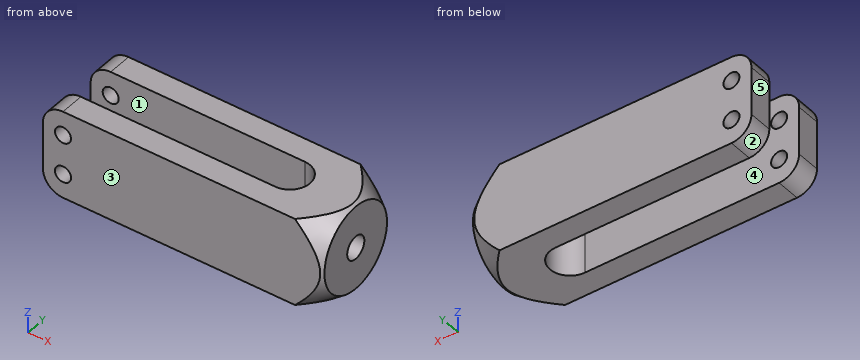
Autodesk Inventor part; units mm, degrees
ref_plane "Work Plane1" through (111.125, 34.925, 0) normal (0, 0.7071, 0.7071) x (-1, 0, 0)
ref_plane "YZ Plane" through (0, 0, 0) normal (1, 0, 0) x (0, 1, 0)
ref_plane "XZ Plane" through (0, 0, 0) normal (0, 1, 0) x (-1, 0, 0)
sketch "Sketch1" plane through (0, 0, 0) normal (0, 0, 1) x (1, 0, 0)
  line L0 (0, 0) -> (111.125, 0)
  line L1 (111.125, 0) -> (111.125, 34.925)
  line L2 (111.125, 34.925) -> (0, 34.925)
  arc A0 (85.0138, 9.525) -> (85.0138, 25.4) centre (85.0138, 17.4625) ccw
  line L3 (85.0138, 25.4) -> (0, 25.4)
  line L4 (0, 9.525) -> (85.0138, 9.525)
  line L5 (85.0138, 9.525) -> (85.0138, 25.4)
  line L6 (0, 34.925) -> (0, 25.4)
  line L7 (0, 9.525) -> (0, 0)
  dimension "d0" = 34.925
  dimension "d2" = 15.875
  dimension "d3" = 85.0138
  dimension "d4" = 111.125
extrude "Extrusion1" add sketch "Sketch1" along normal blind 34.925 contours L7 L4 A0 L3 L6 L2 L1 L0
sketch "Sketch2" plane through (111.125, 0, 0) normal (1, 0, 0) x (0, 0, -1)
  point P0 (0, 0)
  point P1 (-17.4625, 17.4752)
hole "Hole1" at (111.125, 17.4752, 17.4625) direction (-1, 0, 0) diameter 9.144 end through all
ref_plane "Work Plane1" through (111.125, 34.925, 0) normal (0, 0.7071, 0.7071) x (-1, 0, 0)
sketch "Sketch3" plane through (111.125, 34.925, 0) normal (0, 0.7071, 0.7071) x (-1, 0, 0)
  line L0 (0, 0) -> (111.125, 0)
  line L1 (111.125, 0) -> (111.125, 24.6957)
  line L2 (0, 24.6957) -> (111.125, 24.6957)
  line L3 (0, 0) -> (0, 24.6957)
  line L4 (0, 0) -> (0, 24.6957)
  line L5 (0, 8.027) -> (11.1125, 0)
  line L6 (11.1125, 0) -> (0, 0)
  line L7 (0, 8.027) -> (0, 0)
  dimension "d14" = 11.1125
  dimension "d15" = 16.6687
revolve "Revolution1" cut sketch "Sketch3" angle 360 about axis through (111.125, 17.4625, 17.4625) along (-1, 0, 0) contours L3 L5 L0
fillet "Fillet1" radius 7.9375 4 edges at (0, 30.1625, 0) (0, 4.7625, 0) (0, 4.7625, 34.925) (0, 30.1625, 34.925)
sketch "Sketch4" plane through (7.9375, 0, 0) normal (0, -1, 0) x (1, 0, 0)
  point P0 (-7.9375, 0)
  point P1 (0, 9.525)
  point P2 (0, 25.4)
sketch "Sketch5" plane through (7.9375, 34.925, 0) normal (0, 1, 0) x (1, 0, 0)
  line L0 (92.075, -34.925) -> (0, -34.925)
  line L1 (92.075, 0) -> (0, 0)
  point P0 (-7.9375, 0)
  dimension "d18" = 34.925
sketch "Sketch6" plane through (7.9375, 34.925, 0) normal (0, 1, 0) x (1, 0, 0)
  point P0 (-7.9375, 0)
  point P1 (0, -9.525)
  point P2 (0, -25.4)
hole "Hole2" at (7.9375, 34.925, 9.525) direction (0, -1, 0) diameter 6.4008 depth 83.2612 tip angle 118
thread "Thread1"
sketch "Sketch7" plane through (7.9375, 34.925, 0) normal (0, 1, 0) x (1, 0, 0)
  point P0 (-7.9375, 0)
  point P1 (0, -25.4)
hole "Hole3" at (7.9375, 34.925, 25.4) direction (0, -1, 0) diameter 6.35 end through all
properties part number "middle handle piece (hard) (1)" material "Aluminum 6061"
Geometry check sheet. Reference: the model listing, model coordinates, mm. Face numbers are marked on the shaded views. A direction names the side the tool comes from. Coordinates: 2 decimals unless noted, no trailing zeros. Write each loop counter-clockwise with the first axis right and the second up, starting at its lowest first coordinate (ties: lowest second). Pieces come first, ordered by that corner, then holes. Notation, with made-up numbers: M 0.5,-25.75 L 38.5,-25.75 A18 cw 38.5,7.25 Z; hole C -2.75,66.5 d8. An arc over 180 degrees is marked long. Use one line per item in the form item = value. Start each with the question number.
1) Section check A-A on x = 45. Enter the section's corners in (y, z) (3 decimals), and give its area (3 significant figures).
2) Release check for a two-part mould opening along Y. For the marked faces 1, 2 and 3 record: pulls with the +Y half, pulls with the -Y half, needs draft (parallel to the pull), parting line crosses it, or undercut.
3) Set-up check for the marked faces 4 and 5: record each of +Z, -Z, +X, -X, +Y, -Y from which the full face is reachable in a straight line by a thin tool's end or side.
4) Section check D-D on x = 89. Enter the section's corners in (y, z) (3 decimals), and give its area (3 significant figures).
5) Thickness scan on probe 1 along Y at (x, z) = (60.5, 29) (3 decimals); probe 2 along Z at (x, y) = (9.5, 29.5) (3 decimals); probe 3 along X at (y, z) = (26.5, 26) (3 decimals). Record the ranges inside material, lowest first. Write a range as from..to.
6) Section check B-B on z = 25.4. State how many separate pieces and enclosed holes the cut face has, and give its area (3 significant figures).
Responses:
q1.outline = M 0,0 L 9.525,0 L 9.525,34.925 L 0,34.925 Z; M 25.4,0 L 34.925,0 L 34.925,34.925 L 25.4,34.925 Z
q1.area = 665 mm2
q2.face_1 = undercut
q2.face_2 = needs draft
q2.face_3 = pulls with the -Y half
q3.face_4 = +Z, -Z, -X
q3.face_5 = +Z, -Z, -X, +Y, -Y
q4.outline = M 0,0 L 10.599,0 L 10.599,34.925 L 0,34.925 Z; M 24.326,0 L 34.925,0 L 34.925,34.925 L 24.326,34.925 Z
q4.area = 740 mm2
q5.probe_1 = 0..9.525, 25.4..34.925
q5.probe_2 = 0..6.732, 12.318..22.636, 28.164..34.925
q5.probe_3 = 0..4.82, 11.055..111.125
q6.separate_pieces = 3
q6.enclosed_holes = 0
q6.area = 2,300 mm2
